Input: part model. Units: mm. Frame: model coordinates. A direction names the side the tool comes from. Coordinates: 2 decimals unless noted, no trailing zeros. Write each loop counter-clockwise with the first axis right and the second up, starting at its lowest first coordinate (ties: lowest second). Pieces come first, ordered by that corner, then holes. Notation, with made-up numbers: (-32.5, 51) - (-20.5, 51) arc R15 cw to (-20.5, 73) - close; hole circle Ø11 at (-21.75, 87). An arc over 180 degrees is marked (long way). One line per question, with ' | ' between items. Start each with the question number.
1) Section query D-D on y = -11.75. Return loops of the section in (x, z), and give its area (3 significant figures).
2) Section query C-C on y = -1.5. Give the number of separate pieces and of enclosed holes in the cut face, and give its area (3 significant figures).
3) Section query B-B on x = -7. Return loops of the section in (y, z).
4) Draft query along X for faces 1 (the cylindrical face through (-7.189, -9.563, 4.294)), 2 (the cylindrical face through (33, -2, 0)). Return one class per face: released by +X, released by -X, zero draft, split by the parting line, or undercut.
5) Reachability of faces 3 (the flat face through (-11, -2, 1)), 4 (the cylindrical face through (-10.9, -0.99, -0.07)), 5 (the flat face through (25, -1, -3.3)) from +Z, -Z, +X, -X, +Y, -Y: full face, straight path, thin tool, end or side. Return the list, or none.
6) Line query: line 1 (X direction, y = -13, z = 11.5); line 2 (X direction, y = -1.5, z = 2); line 3 (Y direction, x = 17, z = 0.5). Output: solid intervals per line, ascending.
7) First-contact query: P1, Ø5, axis at x = 24, z = -0.5, coming from the +Y side; P2, Ø3, axis at x = -12.5, z = 0, coming from the +Y side; P3, Ø1.5, axis at x = 11.5, z = -6.5, coming from the -Y side; P4, Ø4, axis at x = -10.5, y = -9.5, coming from the -Z side. Flat tips, straight axial feed; report the tip coordinate or a pass-through.
8) Section query A-A on x = 2.5. Return loops of the section in (y, z), and give its area (3 significant figures).
```python
from build123d import *

# Parameters (mm, degrees)
EXTRUDE_1_DEPTH             = 5
EXTRUDE_2_DEPTH             = 9
CUT_EXTRUDE_1_DEPTH         = 1
HOLE_WIZARD_3_0_3_1_D       = 3
HOLE_WIZARD_3_0_3_1_DEPTH   = 3.5
HOLE_WIZARD_3_0_3_1_TIP     = 0.901290929
HOLE_WIZARD_3_0_3_2_D       = 3
HOLE_WIZARD_3_0_3_2_DEPTH   = 3.5
HOLE_WIZARD_3_0_3_2_TIP     = 0.901290929
HOLE_WIZARD_M31_D           = 3.2
HOLE_WIZARD_M31_CBORE_D     = 6.05
HOLE_WIZARD_M31_CBORE_DEPTH = 3
HOLE_WIZARD_16_0_16_1_D     = 16
HOLE_WIZARD_16_0_16_1_DEPTH = 14
HOLE_WIZARD_3_2_3_2_1_D     = 3.2
HOLE_WIZARD_6_0_6_1_D       = 6
HOLE_WIZARD_6_0_6_1_DEPTH   = 13
FILLET_1_R                  = 2
FILLET_2_R                  = 3


with BuildPart() as part:
    # Эскиз1 → Бобышка-Вытянуть1 (new body)
    with BuildSketch(Plane.XZ):
        with BuildLine():
            Line((6.12, -15.860189154), (27.88, -7.463618425))
            ThreePointArc((27.88, -7.463618425), (33, 0), (27.88, 7.463618425))
            Line((27.88, 7.463618425), (6.12, 15.860189154))
            ThreePointArc((6.12, 15.860189154), (-17, 0), (6.12, -15.860189154))
        make_face()
    extrude(amount=-EXTRUDE_1_DEPTH)

    # Эскиз2 → Бобышка-Вытянуть2 (add)
    with BuildSketch(Plane(origin=(0, 5, 0), x_dir=(-1, 0, 0), z_dir=(0, 1, 0))):
        with BuildLine():
            Line((12.124355653, 4), (-12.124355653, 4))
            ThreePointArc((-12.124355653, 4), (-14.722431864, 5.5), (-14.722431864, 8.5))
            ThreePointArc((-14.722431864, 8.5), (0, 17), (14.722431864, 8.5))
            ThreePointArc((14.722431864, 8.5), (14.722431864, 5.5), (12.124355653, 4))
        make_face()
    extrude(amount=EXTRUDE_2_DEPTH)

    # Эскиз3 → Вырез-Вытянуть1 (cut)
    with BuildSketch(Plane.XZ):
        with BuildLine():
            Line((21.85, 3.882975663), (21.85, -3.882975663))
            ThreePointArc((21.85, -3.882975663), (25, -5), (28.15, -3.882975663))
            Line((28.15, -3.882975663), (28.15, 3.882975663))
            ThreePointArc((28.15, 3.882975663), (25, 5), (21.85, 3.882975663))
        make_face()
    extrude(amount=-CUT_EXTRUDE_1_DEPTH, mode=Mode.SUBTRACT)

    # Диаметр отверстия Ø3.0 (3)1
    with Locations(Plane(origin=(0, 0, 0), x_dir=(-1, 0, 0), z_dir=(0, -1, 0))):
        with Locations((0, 12.5)):
            Hole(HOLE_WIZARD_3_0_3_1_D / 2, depth=HOLE_WIZARD_3_0_3_1_DEPTH)
            with Locations((0, 0, -(HOLE_WIZARD_3_0_3_1_DEPTH + HOLE_WIZARD_3_0_3_1_TIP / 2))):  # 118° drill point
                Cone(0, HOLE_WIZARD_3_0_3_1_D / 2, HOLE_WIZARD_3_0_3_1_TIP, mode=Mode.SUBTRACT)

    # Диаметр отверстия Ø3.0 (3)2
    with Locations(Plane(origin=(0, 0, 0), x_dir=(-1, 0, 0), z_dir=(0, -1, 0))):
        with Locations((0, -12.5)):
            Hole(HOLE_WIZARD_3_0_3_2_D / 2, depth=HOLE_WIZARD_3_0_3_2_DEPTH)
            with Locations((0, 0, -(HOLE_WIZARD_3_0_3_2_DEPTH + HOLE_WIZARD_3_0_3_2_TIP / 2))):  # 118° drill point
                Cone(0, HOLE_WIZARD_3_0_3_2_D / 2, HOLE_WIZARD_3_0_3_2_TIP, mode=Mode.SUBTRACT)

    # Цековка для винта с заклепочной головкой M31 (through all)
    with Locations(Plane(origin=(0, 5, 0), x_dir=(1, 0, 0), z_dir=(0, 1, 0))):
        with Locations((12.5, 0), (6.25, 10.825317547), (-6.25, 10.825317547), (-12.5, 0)):
            CounterBoreHole(HOLE_WIZARD_M31_D / 2, HOLE_WIZARD_M31_CBORE_D / 2, HOLE_WIZARD_M31_CBORE_DEPTH)

    # Диаметр отверстия Ø16.0 (16)1
    with Locations(Plane(origin=(0, 0, 0), x_dir=(-1, 0, 0), z_dir=(0, -1, 0))):
        with Locations((0, 0)):
            Hole(HOLE_WIZARD_16_0_16_1_D / 2, depth=HOLE_WIZARD_16_0_16_1_DEPTH)

    # Диаметр отверстия Ø3.2 (3.2)1 (through all)
    with Locations(Plane(origin=(0, 0, 0), x_dir=(-1, 0, 0), z_dir=(0, -1, 0))):
        with Locations((6.25, -10.825317547), (-6.25, -10.825317547)):
            Hole(HOLE_WIZARD_3_2_3_2_1_D / 2)

    # Диаметр отверстия Ø6.0 (6)1
    with Locations(Plane(origin=(0, 1, 0), x_dir=(-1, 0, 0), z_dir=(0, -1, 0))):
        with Locations((-25, 0)):
            Hole(HOLE_WIZARD_6_0_6_1_D / 2, depth=HOLE_WIZARD_6_0_6_1_DEPTH)

    # Скругление1
    fillet_1_edges = [part.edges().sort_by_distance(p)[0] for p in [
        (21.85, 0.5, 3.882975663),
        (28.15, 0.5, 3.882975663),
        (28.15, 0.5, -3.882975663),
        (21.85, 0.5, -3.882975663),
    ]]
    fillet(fillet_1_edges, radius=FILLET_1_R)

    # Скругление2
    fillet_2_edges = [part.edges().sort_by_distance(p)[0] for p in [
        (6.92820323, 9.5, 4),
        (-6.92820323, 9.5, 4),
    ]]
    fillet(fillet_2_edges, radius=FILLET_2_R)


with BuildPart() as body_2:
    # Зеркальное отражение1: mirrored copy
    add(part.part.mirror(Plane(origin=(0, 0, 0), x_dir=(0, 0, 1), z_dir=(0, -1, 0))))


solid = body_2.part
```
Answer key:
1) outline: (-14.72, 8.5) arc R3 ccw to (-12.12, 4) - (-8.49, 4) arc R3 ccw to (-6.17, 5.09) arc R8 cw to (6.17, 5.09) arc R3 ccw to (8.49, 4) - (12.12, 4) arc R3 ccw to (14.72, 8.5) arc R17 ccw to start; hole circle Ø3.2 at (-6.25, 10.83); hole circle Ø3.2 at (6.25, 10.83) | area: 253 mm²
2) separate pieces: 1 | enclosed holes: 10 | area: 929 mm²
3) outline: (-14, 4.39) - (-5, 4.39) - (-5, 3.87) - (0, 3.87) - (0, 9.41) - (-14, 9.41) - close; (-14, 12.24) - (0, 12.24) - (0, 15.49) - (-14, 15.49) - close; (-5, -15.49) - (0, -15.49) - (0, -12.24) - (-2, -12.24) - (-2, -13.76) - (-5, -13.76) - close; (-5, -7.89) - (-2, -7.89) - (-2, -9.41) - (0, -9.41) - (0, -3.87) - (-5, -3.87) - close
4) face 1: undercut | face 2: released by +X
5) face 3: -Y | face 4: +Y, -Y | face 5: +Y
6) line 1: -12.52 to -7.7, -4.8 to 4.8, 7.7 to 12.52 | line 2: -16.88 to -7.75, 7.75 to 22.76, 27.24 to 32.75 | line 3: -5 to 0
7) P1: y = 0 | P2: through | P3: y = -5 | P4: z = 4
8) outline: (-14, 7.6) - (0, 7.6) - (0, 16.82) - (-14, 16.82) - close; (-5, -16.82) - (0, -16.82) - (0, -7.6) - (-5, -7.6) - close | area: 175 mm²
